from build123d import *

# Parameters (mm, degrees)
F0_W     = 152.4
F0_H     = 169.731778
F1_DEPTH = 76.2
F2_R     = 65.070277
F3_DEPTH = 76.201
F4_SIZE  = 5.08


with BuildPart() as f1:
    # F0 (on Front) → F1 (new body)
    with BuildSketch(Plane.XZ):
        with Locations((0, 8.5725)):
            Rectangle(F0_W, F0_H)
    extrude(amount=F1_DEPTH)

    # F2 (on face) → F3 (cut, through all)
    with BuildSketch(Plane(origin=(0, 0, 0), x_dir=(-1, 0, 0), z_dir=(0, 1, 0))):
        Circle(F2_R)
    extrude(amount=-F3_DEPTH, mode=Mode.SUBTRACT)

    # F4
    f4_edges = [f1.edges().sort_by_distance(p)[0] for p in [
        (-76.2, 0, 8.5725),
        (0, 0, 93.438389),
        (76.2, 0, 8.5725),
        (0, 0, -76.293389),
        (65.070277, 0, 0),
        (0, -76.2, -76.293389),
        (-76.2, -38.1, -76.293389),
    ]]
    chamfer(f4_edges, length=F4_SIZE)


solid = f1.part
Source: CAD feature listing. Evaluate the final solid. Frame: model axes, mm. Round coordinates to 2 decimals unless told otherwise and drop trailing zeros. Loops run counter-clockwise (first coordinate to the right, second up) from the corner with the lowest first, then second, coordinate; pieces in that order, holes last. Notation, with made-up numbers: (-6, 81.25) -> (43, 81.25) arc R14 ccw to (43, 91.25) -> close; hole circle Ø10 at (-13.5, 66). An arc over 180 degrees is marked (long way). Answer as a JSON object with one key per item and string values. Group by question number.
Q1. Ray query, line 1 (X direction, y = -24, z = 2); line 2 (Z direction, x = 0, y = -37); line 3 (X direction, y = -56.5, z = -33). Return the intervals inside material, ascending. Write a range as from..to.
Q2. Section query B-B (z = 0). Output: boundary loops of the cut face in (x, y), plus the area to 3 significant figures.
Q3. Section query A-A (x = 0). Output: boundary loops of the cut face in (y, z).
Q4. Section query C-C (y = -29). Output: boundary loops of the cut face in (x, z), plus the area to 3 significant figures.
Q5. Mould query, pull axis Z, two halves, no side actions, for faces 1 (the flat face through (-21, 0, 68)), 2 (the flat face through (-73.624, -40.142, -73.789)), 3 (the flat face through (-1.07, -2.5, 90.86)), 4 (the conical face through (14.159, -4.833, -63.764)). Classes: pulls with the +Z half, pulls with the -Z half, needs draft (parallel to the pull), parting line crosses it, or undercut.
Completed:
{
 "1": {"line 1": "-76.2..-65.04, 65.04..76.2", "line 2": "-76.29..-65.07, 65.07..93.44", "line 3": "-76.2..-56.08, 56.08..76.2"},
 "2": {"outline": "(-76.2, -76.2) -> (-65.07, -76.2) -> (-65.07, -5.08) -> (-70.15, 0) -> (-71.12, 0) -> (-76.2, -5.08) -> close; (65.07, -76.2) -> (76.2, -76.2) -> (76.2, -5.08) -> (71.12, 0) -> (70.15, 0) -> (65.07, -5.08) -> close", "area": "1,640 mm²"},
 "3": {"outline": "(-76.2, -71.21) -> (-71.12, -76.29) -> (-5.08, -76.29) -> (0, -71.21) -> (0, -70.15) -> (-5.08, -65.07) -> (-76.2, -65.07) -> close; (-76.2, 65.07) -> (-5.08, 65.07) -> (0, 70.15) -> (0, 88.36) -> (-5.08, 93.44) -> (-76.2, 93.44) -> close"},
 "4": {"outline": "(-76.2, -71.21) -> (-71.12, -76.29) -> (76.2, -76.29) -> (76.2, 93.44) -> (-76.2, 93.44) -> close; hole circle Ø130.14 at (0, 0)", "area": "12,600 mm²"},
 "5": {"face 1": "needs draft", "face 2": "pulls with the -Z half", "face 3": "pulls with the +Z half", "face 4": "undercut"}
}
